```python
from build123d import *

# Parameters (mm, degrees)
SKETCH1_W           = 1415.68
SKETCH1_H           = 829.31
BOSS_EXTRUDE1_DEPTH = 6.35
CUT_EXTRUDE1_REACH  = 1642.715
SKETCH2_W           = 870
SKETCH2_H           = 230
SKETCH2_W_2         = 290
SKETCH2_H_2         = 218


with BuildPart() as part:
    # Sketch1 → Boss-Extrude1 (new body)
    with BuildSketch(Plane(origin=(0, 0, 0), x_dir=(1, 0, 0), z_dir=(0, 1, 0))):
        with Locations((707.84, 414.655)):
            Rectangle(SKETCH1_W, SKETCH1_H)
    extrude(amount=BOSS_EXTRUDE1_DEPTH)

    # Sketch2 → Cut-Extrude1 (cut, up to next)
    with BuildSketch(Plane(origin=(0, 6.35, 0), x_dir=(1, 0, 0), z_dir=(0, 1, 0)), mode=Mode.PRIVATE) as cut_extrude1_sk1:
        with Locations((525, 200)):
            Rectangle(SKETCH2_W, SKETCH2_H)
    cut_extrude1_tool1 = extrude(cut_extrude1_sk1.sketch, amount=-CUT_EXTRUDE1_REACH, mode=Mode.PRIVATE) & part.part
    # Sketch2 → Cut-Extrude1 (cut, up to next)
    with BuildSketch(Plane(origin=(0, 6.35, 0), x_dir=(1, 0, 0), z_dir=(0, 1, 0)), mode=Mode.PRIVATE) as cut_extrude1_sk2:
        Polygon((7, 668.31), (1252, 668.31), (1171, 527.31), (7, 527.31), align=None)
    cut_extrude1_tool2 = extrude(cut_extrude1_sk2.sketch, amount=-CUT_EXTRUDE1_REACH, mode=Mode.PRIVATE) & part.part
    # Sketch2 → Cut-Extrude1 (cut, up to next)
    with BuildSketch(Plane(origin=(0, 6.35, 0), x_dir=(1, 0, 0), z_dir=(0, 1, 0)), mode=Mode.PRIVATE) as cut_extrude1_sk3:
        with Locations((1264.33, 190)):
            Rectangle(SKETCH2_W_2, SKETCH2_H_2)
    cut_extrude1_tool3 = extrude(cut_extrude1_sk3.sketch, amount=-CUT_EXTRUDE1_REACH, mode=Mode.PRIVATE) & part.part
    add(cut_extrude1_tool1.solids().sort_by_distance((525, 6.35, -200))[0], mode=Mode.SUBTRACT)
    add(cut_extrude1_tool2.solids().sort_by_distance((609.476961, 6.35, -598.600162))[0], mode=Mode.SUBTRACT)
    add(cut_extrude1_tool3.solids().sort_by_distance((1264.33, 6.35, -190))[0], mode=Mode.SUBTRACT)


solid = part.part
```
Geometry check sheet. Reference: the model listing, model coordinates, mm. Coordinates: 2 decimals unless noted, no trailing zeros. Loops run counter-clockwise (first coordinate to the right, second up) from the corner with the lowest first, then second, coordinate; pieces in that order, holes last.
Item 1: Sectioned sample at A-A, the plane z = -167. Record the boundary of the cut face in (x, y).
Item 2: Thickness scan on line 1 (Z direction, x = 430, y = 1.5); line 2 (Z direction, x = 1128, y = 1.75); line 3 (X direction, y = 2.25, z = -228). Record the ranges inside material, lowest first.
Item 3: Sectioned sample at B-B, the plane x = 613. Record the boundary of the cut face in (y, z), then the cut area to 3 significant figures.
Item 4: Sectioned sample at C-C, the plane z = -636. Record the boundary of the cut face in (x, y), then the cut area to 3 significant figures.
Item 5: Sectioned sample at D-D, the plane y = 2.5. Record the boundary of the cut face in (x, z).
Item 6: Go/stop test with a flat-tipped pin: pin 1 Ø1.9 at (x, y) = (378, 2) entering from +Z. Record where the tip stops, or that it passes through.
Item 7: Release check for a two-part mould opening along Z. For faces 1 (the face through (698, 6.35, -420)), 2 (the face through (1212.07, 3.22, -598.8)) record: released by +Z, released by -Z, zero draft, split by the parting line, or undercut.
Check result:
1. outline: (0, 0) - (90, 0) - (90, 6.35) - (0, 6.35) - close; (960, 0) - (1119.33, 0) - (1119.33, 6.35) - (960, 6.35) - close; (1409.33, 0) - (1415.68, 0) - (1415.68, 6.35) - (1409.33, 6.35) - close
2. line 1: z = -829.31 to -668.31, -527.31 to -315, -85 to 0
2. line 2: z = -829.31 to -668.31, -527.31 to -299, -81 to 0
2. line 3: x = 0 to 90, 960 to 1119.33, 1409.33 to 1415.68
3. outline: (0, -829.31) - (6.35, -829.31) - (6.35, -668.31) - (0, -668.31) - close; (0, -527.31) - (6.35, -527.31) - (6.35, -315) - (0, -315) - close; (0, -85) - (6.35, -85) - (6.35, 0) - (0, 0) - close
3. area: 2,910 mm2
4. outline: (0, 0) - (7, 0) - (7, 6.35) - (0, 6.35) - close; (1233.44, 0) - (1415.68, 0) - (1415.68, 6.35) - (1233.44, 6.35) - close
4. area: 1,200 mm2
5. outline: (0, -829.31) - (1415.68, -829.31) - (1415.68, 0) - (0, 0) - close; hole (7, -668.31) - (1252, -668.31) - (1171, -527.31) - (7, -527.31) - close; hole (90, -315) - (960, -315) - (960, -85) - (90, -85) - close; hole (1119.33, -299) - (1409.33, -299) - (1409.33, -81) - (1119.33, -81) - close
6. pin 1: stops at z = 0
7. face 1: zero draft
7. face 2: undercut
